Source: CAD feature listing. Evaluate the final solid. Frame: model axes, mm. A direction names the side the tool comes from. Coordinates: 2 decimals unless noted, no trailing zeros. Order: outer loops, then holes, each group sorted by start corner. A loop starts at its lowest first (then second) coordinate and runs counter-clockwise, first axis right, second up. Notation, with made-up numbers: (26.5, 53.5) -> (33.5, 53.5) arc R26 cw to (33.5, 90.5) -> close; hole circle Ø1 at (18.5, 9). An arc over 180 degrees is marked (long way). Put each result on its own line as item: value.
from build123d import *

# Parameters (mm, degrees)
F0_W      = 80
F0_H      = 6
F1_DEPTH  = 15
F4_R      = 2.55
F2_R      = 2.655
F7_D      = 3.5
F8_R      = 2
F9_W      = 5
F9_H      = 1
F10_DEPTH = 0.5


with BuildPart() as f1:
    # F0 (on Top) → F1 (new body)
    with BuildSketch(Plane.XY):
        Rectangle(F0_W, F0_H)
    extrude(amount=F1_DEPTH)

    # F4 (on offset) → F5 section 0
    with BuildSketch(Plane.XZ.offset(-0.8)):
        with Locations((-30, 7.5)):
            Circle(F4_R)
    # F2 (on face) → F5 section 1
    with BuildSketch(Plane.XZ.offset(3)):
        with Locations((-30, 7.5)):
            Circle(F2_R)
    loft(mode=Mode.SUBTRACT)

    # F2 (on face) → F6 section 0
    with BuildSketch(Plane.XZ.offset(3)):
        with Locations((30, 7.5)):
            Circle(F2_R)
    # F4 (on offset) → F6 section 1
    with BuildSketch(Plane.XZ.offset(-0.8)):
        with Locations((30, 7.5)):
            Circle(F4_R)
    loft(mode=Mode.SUBTRACT)

    # F7 (through all)
    with Locations(Plane.XZ.offset(-0.8)):
        with Locations((30, 7.5), (-30, 7.5)):
            Hole(F7_D / 2)

    # F8
    f8_edges = [f1.edges().sort_by_distance(p)[0] for p in [
        (0, -3, 0),
    ]]
    fillet(f8_edges, radius=F8_R)

    # F9 (on face) → F10 (cut)
    with BuildSketch(Plane.XY.offset(15)):
        with Locations((30, 0)):
            Rectangle(F9_W, F9_H)
    extrude(amount=-F10_DEPTH, mode=Mode.SUBTRACT)


solid = f1.part
1. Cut plane C-C on x = -30. Output: boundary loops of the cut face in (y, z) (3 decimals).
Numbers:
outline: (-3, 2) arc R2 ccw to (-1, 0) -> (3, 0) -> (3, 5.75) -> (0.8, 5.75) -> (0.8, 4.95) -> (-3, 4.845) -> close; (-3, 10.155) -> (0.8, 10.05) -> (0.8, 9.25) -> (3, 9.25) -> (3, 15) -> (-3, 15) -> close
2. Pull-direction query (Z, two-part tool) for faces 1 (the cylindrical face through (31.75, 1.92, 7.58)), 2 (the flat face through (-40, 0, 7)), 3 (the flat face through (-1, 1, 0)); classes: pulls with the +Z half, pulls with the -Z half, needs draft (parallel to the pull), parting line crosses it, or undercut.
Numbers:
face 1: undercut
face 2: needs draft
face 3: pulls with the -Z half
3. First-contact query: pin 1 (4 mm diameter, centred on x = -30, z = 7.5, fed in from -Y). Flat tip, straight axial feed; report the tip coordinate or a pass-through.
Numbers:
pin 1: stops at y = 0.8
4. Ray query, line 1 along Z through (x, y) = (30, 2.2); line 2 along X through (y, z) = (-0.5, 8.25); line 3 along X through (y, z) = (-2.5, 7). Return the intervals inside material, ascending.
Numbers:
line 1: z = 0 to 5.75, 9.25 to 15
line 2: x = -40 to -32.47, -27.53 to 27.53, 32.47 to 40
line 3: x = -40 to -32.59, -27.41 to 27.41, 32.59 to 40
5. Cut plane A-A on x = 30. Output: boundary loops of the cut face in (y, z) (3 decimals), plus the area to 3 significant figures.
Numbers:
outline: (-3, 2) arc R2 ccw to (-1, 0) -> (3, 0) -> (3, 5.75) -> (0.8, 5.75) -> (0.8, 4.95) -> (-3, 4.845) -> close; (-3, 10.155) -> (0.8, 10.05) -> (0.8, 9.25) -> (3, 9.25) -> (3, 15) -> (0.5, 15) -> (0.5, 14.5) -> (-0.5, 14.5) -> (-0.5, 15) -> (-3, 15) -> close
area: 61.2 mm2
6. Set-up query: faces 4 (the cylindrical face through (-28.25, 1.92, 7.58)), 5 (the conical face through (29.66, -1.07, 10.08)). Return all of +Z, -Z, +X, -X, +Y, -Y with unobstructed straight access to the full face (end or side cutting, diameter ignored); none if empty.
Numbers:
face 4: +Y, -Y
face 5: -Y
7. Cut plane B-B on y = 2. Output: boundary loops of the cut face in (x, z).
Numbers:
outline: (-40, 0) -> (40, 0) -> (40, 15) -> (-40, 15) -> close; hole circle Ø3.5 at (-30, 7.5); hole circle Ø3.5 at (30, 7.5)
8. Cut plane D-D on z = 7.5. Count the separate pieces of the cut face and the enclosed holes in it, plus the area to 3 significant figures.
Numbers:
separate pieces: 3
enclosed holes: 0
area: 425 mm2
